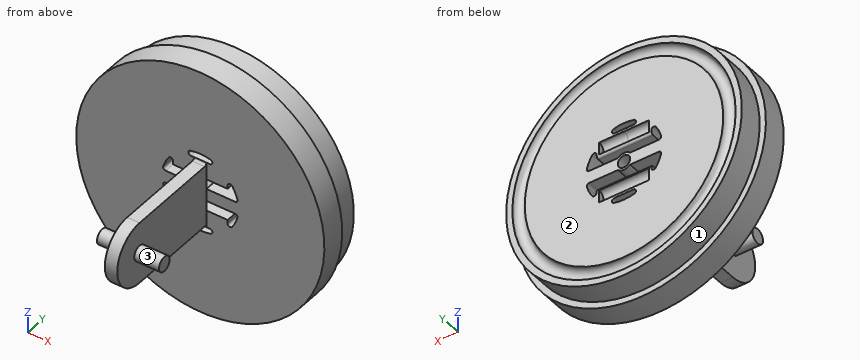
from build123d import *

# Parameters (mm, degrees)
SKETCH1_R           = 50
BOSS_EXTRUDE1_DEPTH = 10
SKETCH3_R           = 47.5
BOSS_EXTRUDE2_DEPTH = 10
SKETCH5_R           = 2.5
SKETCH6_R           = 2.5
CUT_EXTRUDE1_DEPTH  = 5
CUT_EXTRUDE2_START  = -0.01
SKETCH7_R           = 47.5
CUT_EXTRUDE2_DEPTH  = 0.01
SKETCH10_R          = 2.5
CUT_EXTRUDE4_DEPTH  = 10
CUT_EXTRUDE7_DEPTH  = 74.481971258
FILLET1_R           = 1
FILLET2_R           = 1
BOSS_EXTRUDE3_DEPTH = 2.5
FILLET3_R           = 1
FILLET4_START       = -12
FILLET4_DEPTH       = 24
FILLET5_R           = 1
SKETCH14_R          = 3
BOSS_EXTRUDE5_DEPTH = 10


with BuildPart() as part:
    # Sketch1 → Boss-Extrude1 (new body)
    with BuildSketch(Plane(origin=(0, 0, 0), x_dir=(1, 0, 0), z_dir=(0, 1, 0))):
        with Locations(Location((0, 0, 0), (0, 0, 270))):
            Circle(SKETCH1_R)
    extrude(amount=BOSS_EXTRUDE1_DEPTH)

    # Sketch3 → Boss-Extrude2 (add)
    with BuildSketch(Plane(origin=(0, 10, 0), x_dir=(1, 0, 0), z_dir=(0, 1, 0))):
        with Locations(Location((0, 0, 0), (0, 0, 270))):
            Circle(SKETCH3_R)
    extrude(amount=BOSS_EXTRUDE2_DEPTH)

    # Cut-Sweep1: sweep along a path in Sketch4
    with BuildLine(Plane(origin=(0, 20, 0), x_dir=(1, 0, 0), z_dir=(0, 1, 0))) as cut_sweep1_path:
        CenterArc((0, 0), 42.5, 0, 360)
    # Sketch5 → Cut-Sweep1 (sweep, cut)
    with BuildSketch(Plane.XY):
        with Locations((42.5, 20)):
            Circle(SKETCH5_R)
    sweep(path=cut_sweep1_path.line, mode=Mode.SUBTRACT)

    # Sketch6 → Cut-Extrude1 (cut)
    with BuildSketch(Plane(origin=(0, 20, 0), x_dir=(1, 0, 0), z_dir=(0, 1, 0))):
        with Locations(Location((0, 0, 0), (0, 0, 270))):
            Circle(SKETCH6_R)
    extrude(amount=-CUT_EXTRUDE1_DEPTH, mode=Mode.SUBTRACT)

    # Sketch7 → Cut-Extrude2 (cut)
    with BuildSketch(Plane(origin=(0, 20, 0), x_dir=(1, 0, 0), z_dir=(0, 1, 0)).offset(CUT_EXTRUDE2_START)):
        with Locations(Location((0, 0, 0), (0, 0, 270))):
            Circle(SKETCH7_R)
    extrude(amount=CUT_EXTRUDE2_DEPTH, mode=Mode.SUBTRACT)

    # Sketch10 → Cut-Extrude4 (cut, symmetric)
    with BuildSketch(Plane(origin=(0, 0, 0), x_dir=(0, 0, -1), z_dir=(1, 0, 0))):
        with Locations((-10, 19.99)):
            Circle(SKETCH10_R)
        with Locations((10, 19.99)):
            Circle(SKETCH10_R)
    extrude(amount=CUT_EXTRUDE4_DEPTH, both=True, mode=Mode.SUBTRACT)

    # Sketch11 → Cut-Extrude7 (cut, through all)
    with BuildSketch(Plane(origin=(0, 19.99, 0), x_dir=(1, 0, 0), z_dir=(0, 1, 0))):
        with BuildLine():
            ThreePointArc((-2.449489743, 2.5), (0, 3.5), (2.449489743, 2.5))
            Line((2.449489743, 2.5), (15.209986881, 2.5))
            ThreePointArc((15.209986881, 2.5), (13.746070636, 6.974184039), (11, 10.797856312))
            Line((11, 10.797856312), (11, 6.5))
            Line((11, 6.5), (-11, 6.5))
            Line((-11, 6.5), (-11, 10.797856312))
            ThreePointArc((-11, 10.797856312), (-13.746070636, 6.974184039), (-15.209986881, 2.5))
            Line((-15.209986881, 2.5), (-2.449489743, 2.5))
        make_face()
        with BuildLine():
            ThreePointArc((11, -10.797856312), (13.746070636, -6.974184039), (15.209986881, -2.5))
            Line((15.209986881, -2.5), (2.449489743, -2.5))
            ThreePointArc((2.449489743, -2.5), (0, -3.5), (-2.449489743, -2.5))
            Line((-2.449489743, -2.5), (-15.209986881, -2.5))
            ThreePointArc((-15.209986881, -2.5), (-13.746070636, -6.974184039), (-11, -10.797856312))
            Line((-11, -10.797856312), (-11, -6.5))
            Line((-11, -6.5), (11, -6.5))
            Line((11, -6.5), (11, -10.797856312))
        make_face()
        with BuildLine():
            ThreePointArc((-8.587782019, -13.5), (0, -16), (8.587782019, -13.5))
            Line((8.587782019, -13.5), (-8.587782019, -13.5))
        make_face()
        with BuildLine():
            Line((-8.587782019, 13.5), (8.587782019, 13.5))
            ThreePointArc((8.587782019, 13.5), (0, 16), (-8.587782019, 13.5))
        make_face()
    extrude(amount=-CUT_EXTRUDE7_DEPTH, mode=Mode.SUBTRACT)

    # Fillet1
    fillet1_edges = [part.edges().sort_by_distance(p)[0] for p in [
        (11, 9.995, 10.797856312),
        (-11, 9.995, 10.797856312),
        (-15.209986881, 9.995, 2.5),
        (15.209986881, 9.995, 2.5),
        (15.209986881, 9.995, -2.5),
        (-15.209986881, 9.995, -2.5),
        (-11, 9.995, -10.797856312),
        (11, 9.995, -10.797856312),
    ]]
    fillet(fillet1_edges, radius=FILLET1_R)

    # Fillet2
    fillet2_edges = [part.edges().sort_by_distance(p)[0] for p in [
        (-8.587782019, 9.995, -13.5),
        (8.587782019, 9.995, -13.5),
        (8.587782019, 9.995, 13.5),
        (-8.587782019, 9.995, 13.5),
    ]]
    fillet(fillet2_edges, radius=FILLET2_R)

    # Sketch13 → Boss-Extrude3 (add, symmetric)
    with BuildSketch(Plane(origin=(0, 0, 0), x_dir=(0, 0, -1), z_dir=(1, 0, 0))):
        with BuildLine():
            Line((-12.5, 0), (12.5, 0))
            Line((12.5, 0), (12.5, -37.5))
            ThreePointArc((12.5, -37.5), (0, -50), (-12.5, -37.5))
            Line((-12.5, -37.5), (-12.5, 0))
        make_face()
    extrude(amount=BOSS_EXTRUDE3_DEPTH, both=True)

    # Fillet3
    fillet3_edges = [part.edges().sort_by_distance(p)[0] for p in [
        (0, 0, -12.5),
        (0, 0, 12.5),
    ]]
    fillet(fillet3_edges, radius=FILLET3_R - 0.0001)  # a hair under: the kernel refuses the full size

    # Fillet4: read off the stored shape, not the designer's step
    # Fillet4 outline → Fillet4 (cut)
    with BuildSketch(Plane.YZ.offset(FILLET4_START)):
        with BuildLine():
            ThreePointArc((18.99, -6.5), (19.697106781, -6.792893219), (19.99, -7.5))
            Line((19.99, -7.5), (19.99, -6.5))
            Line((19.99, -6.5), (18.99, -6.5))
        make_face()
    extrude(amount=FILLET4_DEPTH, mode=Mode.SUBTRACT)

    # Fillet5
    fillet5_edges = [part.edges().sort_by_distance(p)[0] for p in [
        (0, 19.99, 6.5),
    ]]
    fillet(fillet5_edges, radius=FILLET5_R - 0.0001)  # a hair under: the kernel refuses the full size

    # Sketch14 → Boss-Extrude5 (add)
    with BuildSketch(Plane(origin=(2.5, 0, 0), x_dir=(0, 0, -1), z_dir=(1, 0, 0))):
        with Locations((0, -37.5)):
            Circle(SKETCH14_R)
    boss_extrude5 = extrude(amount=BOSS_EXTRUDE5_DEPTH)

    # Mirror2: Boss-Extrude5 across plane
    add(boss_extrude5.mirror(Plane(origin=(0, 0, 0), x_dir=(0, 0, 1), z_dir=(1, 0, 0))))


solid = part.part
Input: part model. Units: mm. Frame: model coordinates. Face numbers are marked on the shaded views. Give positions to 0.01 mm unless a question says otherwise; leave off trailing zeros. Order: outer loops, then holes, each group sorted by start corner. A loop starts at its lowest first (then second) coordinate and runs counter-clockwise, first axis right, second up. Notation, with made-up numbers: (-29, 6) - (17, 6) arc R12 cw to (17, 16) - close; hole circle Ø10 at (-3, -20.5). An arc over 180 degrees is marked (long way). Answer as a JSON object with one key per item and string values. Group by question number.
Q1. Mould query, pull axis Y, two halves, no side actions, for the marked faces 1, 2 and 3. Classes: pulls with the +Y half, pulls with the -Y half, needs draft (parallel to the pull), parting line crosses it, or undercut.
Q2. Cut plane A-A, the plane z = 0. Output: boundary loops of the cut face in (x, y), then the cut area to 3 significant figures.
Q3. Cut plane C-C, the plane y = -45.5. Output: boundary loops of the cut face in (x, z).
Q4. First-contact query: pin 1 Ø3 at (y, z) = (-36, -0.5) entering from -X; pin 2 Ø8 at (x, y) = (-6.5, 0.5) entering from +Z; pin 3 Ø1.6 at (y, z) = (14.5, 7) entering from +X. Flat tips, straight axial feed; report the tip coordinate or a pass-through.
Q5. Line query: probe 1 along X at (y, z) = (17.7, 0); probe 2 along Z at (x, y) = (5, 1.5); probe 3 along X at (y, z) = (16.35, 0). Output: solid intervals per line, ascending.
Q6. Cut plane B-B, the plane y = -20. Output: boundary loops of the cut face in (x, z).
Results:
{
 "1": {"face 1": "needs draft", "face 2": "pulls with the +Y half", "face 3": "undercut"},
 "2": {"outline": "(-50, 0) - (-2.5, 0) - (-2.5, -34.5) - (-12.5, -34.5) - (-12.5, -40.5) - (-2.5, -40.5) - (-2.5, -50) - (2.5, -50) - (2.5, -40.5) - (12.5, -40.5) - (12.5, -34.5) - (2.5, -34.5) - (2.5, 0) - (50, 0) - (50, 10) - (47.5, 10) - (47.5, 19.99) - (45, 19.99) arc R2.5 cw to (40, 19.99) - (2.5, 19.99) - (2.5, 15) - (-2.5, 15) - (-2.5, 19.99) - (-40, 19.99) arc R2.5 cw to (-45, 19.99) - (-47.5, 19.99) - (-47.5, 10) - (-50, 10) - close", "area": "2,270 mm^2"},
 "3": {"outline": "(-2.5, -9.6) - (2.5, -9.6) - (2.5, 9.6) - (-2.5, 9.6) - close"},
 "4": {"pin 1": "x = -12.5", "pin 2": "z = 49.94", "pin 3": "x = 47.09"},
 "5": {"probe 1": "-47.5 to -43.48, -41.52 to -2.5, 2.5 to 41.52, 43.48 to 47.5", "probe 2": "-49.75 to -6.5, -2.5 to 2.5, 6.5 to 49.75", "probe 3": "-47.5 to -2.5, 2.5 to 47.5"},
 "6": {"outline": "(-2.5, -12.5) - (2.5, -12.5) - (2.5, 12.5) - (-2.5, 12.5) - close"}
}
